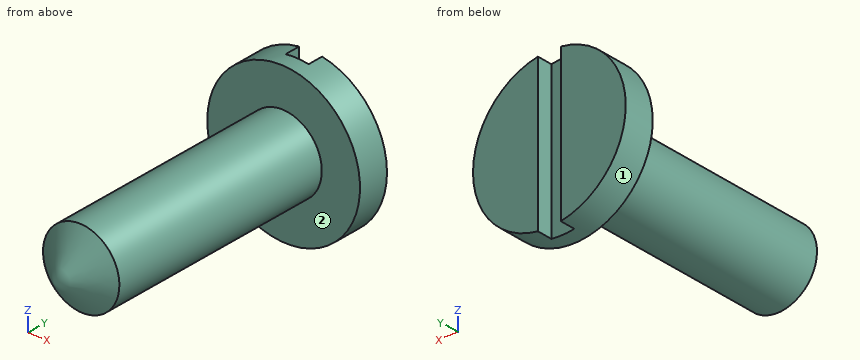
```python
from build123d import *

# Parameters (mm, degrees)
CUT_EXTRUDE1_DEPTH      = 20.241881405
CUT_EXTRUDE1_DEPTH_BACK = 20.241881405
SKETCH2_W               = 1.5
SKETCH2_H               = 1


with BuildPart() as part:
    # Sketch1 → Revolve1 (revolve)
    with BuildSketch(Plane.XY, mode=Mode.PRIVATE) as revolve1_sk:
        Polygon((0, 0), (0, 15), (2.5, 15), (2.5, 17), (-2.5, 17), (-2.5, 0), align=None)
    revolve(revolve1_sk.sketch.rotate(Axis((-2.5, 17, 0), (0, -1, 0)), 180), axis=Axis((-2.5, 17, 0), (0, -1, 0)))

    # Sketch2 → Cut-Extrude1 (cut, two sides: drawn at the far end of the back side and taken through both)
    with BuildSketch(Plane.XY.offset(-CUT_EXTRUDE1_DEPTH_BACK)):
        with Locations((-2.5, 16.5)):
            Rectangle(SKETCH2_W, SKETCH2_H)
    extrude(amount=CUT_EXTRUDE1_DEPTH + CUT_EXTRUDE1_DEPTH_BACK, mode=Mode.SUBTRACT)

    # Sketch3 → Revolve2 (revolve)
    with BuildSketch(Plane.XY, mode=Mode.PRIVATE) as revolve2_sk:
        Polygon((-2.5, 0), (-2.5, -2), (0, 0), align=None)
    revolve(revolve2_sk.sketch.rotate(Axis((-2.5, 0, 0), (0, -1, 0)), 90), axis=Axis((-2.5, 0, 0), (0, -1, 0)))


solid = part.part
```
Source: CAD feature listing. Evaluate the final solid. Frame: model axes, mm. Face numbers are marked on the shaded views. A direction names the side the tool comes from. Round coordinates to 2 decimals unless told otherwise and drop trailing zeros. Loops run counter-clockwise (first coordinate to the right, second up) from the corner with the lowest first, then second, coordinate; pieces in that order, holes last. Notation, with made-up numbers: (-19.5, -33.5) - (26.5, -33.5) arc R16 cw to (26.5, -7.5) - close; hole circle Ø3 at (-11, -17). An arc over 180 degrees is marked (long way). Use CSV: the item, a comma, the result in double quotes.
Q1. Pin query (flat end, axial travel): pin 1 Ø2 at (y, z) = (14.5, 1.5) entering from +X; pin 2 Ø0.8 at (y, z) = (16.5, -1.5) entering from +X; pin 3 Ø5 at (x, y) = (-3.5, 2.5) entering from +Z. Return the tip coordinate at first contact, or that it passes through.
Reported:
pin 1,"x = 2.46"
pin 2,"x = 2.38"
pin 3,"z = 2.5"
Q2. Section query C-C, the plane x = -5.25. Output: boundary loops of the cut face in (y, z).
Reported:
outline,"(15, -4.18) - (17, -4.18) - (17, 4.18) - (15, 4.18) - close"
Q3. Ray query, line 1 along Y through (x, z) = (1.25, -1.5); line 2 along Z through (x, y) = (-4.25, 15.5); line 3 along Z through (x, y) = (0.5, 15.25). Return the intervals inside material, ascending.
Reported:
line 1,"15 to 17"
line 2,"-4.68 to 4.68"
line 3,"-4 to 4"
Q4. Section query A-A, the plane y = 13.75. Output: boundary loops of the cut face in (x, z).
Reported:
outline,"circle Ø5 at (-2.5, 0)"
Q5. Section query B-B, the plane x = -6.5. Output: boundary loops of the cut face in (y, z), then the cut area to 3 significant figures.
Reported:
outline,"(15, -3) - (17, -3) - (17, 3) - (15, 3) - close"
area,"12.0 mm^2"
Q6. Reachability of the marked faces 1 and 2 from +Z, -Z, +X, -X, +Y, -Y: full face, straight path, thin tool, end or side. Return the list, or none.
Reported:
face 1,"+Y, -Y"
face 2,"-Y"
